from build123d import *

# Parameters (mm, degrees)
SKETCH1_W           = 12
SKETCH1_H           = 27
BOSS_EXTRUDE1_DEPTH = 3
SKETCH2_W           = 12
SKETCH2_H           = 2
BOSS_EXTRUDE2_DEPTH = 9
SKETCH3_R           = 2.5
CUT_EXTRUDE1_DEPTH  = 10
SKETCH4_R           = 1.2
CUT_EXTRUDE2_DEPTH  = 10
SKETCH5_R           = 1.2
CUT_EXTRUDE3_DEPTH  = 10


with BuildPart() as part:
    # Sketch1 → Boss-Extrude1 (new body)
    with BuildSketch(Plane.XY):
        with Locations((6, 13.5)):
            Rectangle(SKETCH1_W, SKETCH1_H)
    extrude(amount=BOSS_EXTRUDE1_DEPTH)

    # Sketch2 → Boss-Extrude2 (add)
    with BuildSketch(Plane.XY.offset(3)):
        with Locations((6, 1)):
            Rectangle(SKETCH2_W, SKETCH2_H)
    extrude(amount=BOSS_EXTRUDE2_DEPTH)

    # Sketch3 → Cut-Extrude1 (cut)
    with BuildSketch(Plane(origin=(0, 2, 0), x_dir=(1, 0, 0), z_dir=(0, 1, 0))):
        with Locations((6, -7)):
            Circle(SKETCH3_R)
    extrude(amount=-CUT_EXTRUDE1_DEPTH, mode=Mode.SUBTRACT)

    # Sketch4 → Cut-Extrude2 (cut)
    with BuildSketch(Plane.XY.offset(3)):
        with Locations((9.236141261, 11.9)):
            Circle(SKETCH4_R)
        with Locations((9.236141261, 21.8)):
            Circle(SKETCH4_R)
    extrude(amount=-CUT_EXTRUDE2_DEPTH, mode=Mode.SUBTRACT)

    # Sketch5 → Cut-Extrude3 (cut)
    with BuildSketch(Plane.XY.offset(3)):
        with Locations((6.752182316, 11.9)):
            Circle(SKETCH5_R)
        with Locations((6.752182316, 21.8)):
            Circle(SKETCH5_R)
    extrude(amount=-CUT_EXTRUDE3_DEPTH, mode=Mode.SUBTRACT)


solid = part.part
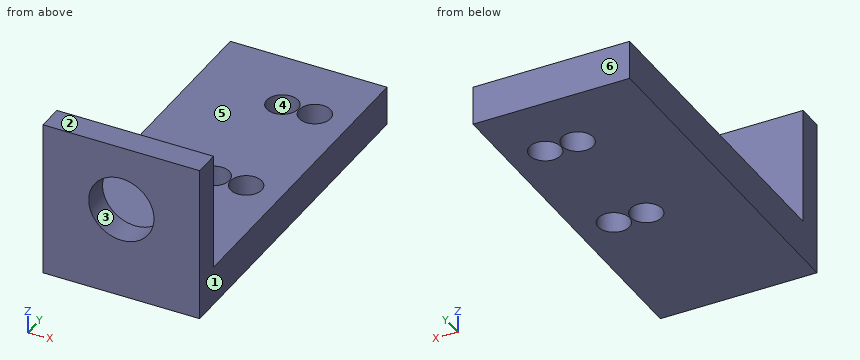
Check sheet for the modelled part. Datum: model origin and axes. Units: mm. Face numbers are marked on the shaded views. A direction names the side the tool comes from. Give positions to 0.01 mm unless a question says otherwise; leave off trailing zeros. Write each loop counter-clockwise with the first axis right and the second up, starting at its lowest first coordinate (ties: lowest second). Pieces come first, ordered by that corner, then holes. Notation, with made-up numbers: (22, 48.25) -> (51, 48.25) arc R20 ccw to (51, 78.25) -> close; hole circle Ø4 at (19, 11). An arc over 180 degrees is marked (long way). Use one line per item in the form item = value. Start each with the question number.
1. Access from +Z, -Z, +X, -X, +Y, -Y to the whole of each face (thin tool, end or side, straight path). Record for the marked faces 5 and 6.
2. Section check C-C (x = 6). Record the cut outline in (y, z) (3 decimals), and give its area (3 significant figures).
3. Mould release check, pull along X, two halves, no side actions. Record for the marked faces 1, 2, 3 and 4: pulls with the +X half, pulls with the -X half, needs draft (parallel to the pull), parting line crosses it, or undercut.
4. Section check D-D (x = 1.5). Record the cut outline in (y, z).
5. Go/stop test with flat-tipped pins: P1, Ø6, axis at x = 4.5, z = 7.5, coming from the +Y side; P2, Ø4, axis at x = 4, y = 14.5, coming from the +Z side. Record where each tip stops, or that it passes through.
6. Thickness scan on line 1 along X through (y, z) = (1.65, 7); line 2 along Z through (x, y) = (6, 1.3); line 3 along Z through (x, y) = (8.5, 18). Record the ranges inside material, lowest first. Write a range as from..to.
7. Section check B-B (y = 11.9). Record the cut outline in (x, z).
8. Section check A-A (z = 7). Record the cut outline in (x, y), and give its area (3 significant figures).
Conclusion:
q1.face_5 = +Z, +X, -X, +Y
q1.face_6 = +Z, -Z, +X, -X, +Y
q2.outline = (0, 0) -> (10.965, 0) -> (10.965, 3) -> (2, 3) -> (2, 4.5) -> (0, 4.5) -> close; (0, 9.5) -> (2, 9.5) -> (2, 12) -> (0, 12) -> close; (12.835, 0) -> (20.865, 0) -> (20.865, 3) -> (12.835, 3) -> close; (22.735, 0) -> (27, 0) -> (27, 3) -> (22.735, 3) -> close
q2.area = 77.8 mm²
q3.face_1 = pulls with the +X half
q3.face_2 = needs draft
q3.face_3 = undercut
q3.face_4 = undercut
q4.outline = (0, 0) -> (27, 0) -> (27, 3) -> (2, 3) -> (2, 12) -> (0, 12) -> close
q5.P1 = 2
q5.P2 = 3
q6.line_1 = 0..3.5, 8.5..12
q6.line_2 = 0..4.5, 9.5..12
q6.line_3 = 0..3
q7.outline = (0, 0) -> (5.55, 0) -> (5.55, 3) -> (0, 3) -> close; (7.95, 0) -> (8.04, 0) -> (8.04, 3) -> (7.95, 3) -> close; (10.44, 0) -> (12, 0) -> (12, 3) -> (10.44, 3) -> close
q8.outline = (0, 0) -> (3.5, 0) -> (3.5, 2) -> (0, 2) -> close; (8.5, 0) -> (12, 0) -> (12, 2) -> (8.5, 2) -> close
q8.area = 14.0 mm²
